Read the model definition and answer for the solid it produces. Units are mm, in the model's axes. A direction names the side the tool comes from. Give positions to 0.01 mm unless a question says otherwise; leave off trailing zeros. Write each loop counter-clockwise with the first axis right and the second up, starting at its lowest first coordinate (ties: lowest second). Pieces come first, ordered by that corner, then holes. Notation, with made-up numbers: M -28,20 L 5,20 A16 cw 5,49 Z; hole C 74,41 d3. An arc over 180 degrees is marked long. Use a Markdown table: item, result. Add a question column.
Item 1: A cutting plane is placed at A-A on x = -59.5. Determine the outline of the cut face in (y, z).
Item 2: For faces 1 (the flat face through (-43.365, -85.368, -12.86)), 2 (the cylindrical face through (-69.5, -93.5, -24.5)), determine the directions among +Z, -Z, +X, -X, +Y, -Y from which every point of the face is accessible in a straight line to the end or side of a thin tool.
Item 3: A cutting plane is placed at B-B on z = -5.75. Determine the outline of the cut face in (x, y), then the cut area to 3 significant figures.
Item 4: Consider probe 1 along Z at (x, y) = (-61, -96); probe 2 along Y at (x, z) = (-68.5, -18.25); probe 3 along Y at (x, z) = (-72, -5.25). Determine where each line is inside the solid, lowest interval first. Write a range as [from, to].
Item 5: A cutting plane is placed at C-C on y = -65.5. Determine the outline of the cut face in (x, z).
Item 6: Given P1, Ø6, axis at y = -72, z = -7, coming from the -X side; P2, Ø10, axis at x = -63.5, y = -90, coming from the +Z side; P3, Ø6, axis at x = -56.5, z = -17.5, coming from the -Y side; P4, Ø10, axis at x = -44, z = -18.5, coming from the -Y side, each flat-ended and moving along its own axis, determine where each tip first touches the part or whether it passes through.
Item 7: A cutting plane is placed at D-D on x = -68. Count the separate pieces of the cut face and the enclosed holes in it, then the cut area to 3 significant figures.
Item 8: The mould has two halves that part along Z. Classify faces 3 (the flat face through (-50, -90, -26)), 4 (the flat face through (-46.063, -70.681, -12.86)), 5 (the flat face through (-48.637, -69.14, -12.818)): pulls with the +Z half, pulls with the -Z half, needs draft (parallel to the pull), parting line crosses it, or undercut.
Autodesk Inventor part; units mm, degrees
ref_plane "YZ Plane" through (0, 0, 0) normal (1, 0, 0) x (0, 1, 0)
ref_plane "XZ Plane" through (0, 0, 0) normal (0, 1, 0) x (-1, 0, 0)
ref_plane "XY Plane" through (0, 0, 0) normal (0, 0, 1) x (1, 0, 0)
sketch "Sketch1" plane through (0, 0, 0) normal (0, 0, 1) x (1, 0, 0)
  circle A0 centre (-48.3826, -94.0192) radius 2.5
  circle A1 centre (2.8152, 8.6005) radius 2.5
  line L0 (-48.3826, -94.0192) -> (40.5013, 54.4144)
  line L1 (2.8152, 8.6005) -> (32.8522, -42.034)
  line L2 (-2.0828, 38.9998) -> (-2.0828, -39)
  line L3 (-2.0828, -0.0001) -> (69.8745, -0.0001)
  line L4 (7.9172, -0.0001) -> (-0.6834, -5.1021)
  line L5 (2.8152, 8.6005) -> (7.9172, -0.0001)
  line L6 (7.9172, -0.0001) -> (16.5177, 5.1019)
  line L7 (7.9172, -0.0001) -> (-0.6834, -5.1021)
  line L8 (-0.6834, -5.1021) -> (-0.6834, -5.1021)
  line L9 (7.9172, -0.0001) -> (16.5177, 5.1019)
  line L10 (16.5177, 5.1019) -> (16.5177, 5.1019)
  line L11 (7.9172, -0.0001) -> (-0.6622, 5.1374)
  line L12 (7.9172, -0.0001) -> (16.4966, -5.1375)
  line L13 (-48.3826, -94.0192) -> (-43.2452, -85.4397)
  line L14 (-54.6233, -56.9895) -> (-9.7188, -83.8789)
  line L15 (-43.2452, -85.4397) -> (-34.6657, -90.5772)
  line L16 (-43.2452, -85.4397) -> (-51.8246, -80.3023)
  line L17 (-34.6657, -90.5772) -> (16.4966, -5.1375)
  line L18 (-0.6622, 5.1374) -> (-51.8246, -80.3023)
  line L19 (-3.7386, 0) -> (13.452, 10.2217)
  line L20 (-3.7386, 0) -> (13.4203, -10.2749)
  circle A2 centre (6.9172, -34) radius 2.5
  circle A3 centre (6.9172, -34) radius 5
  circle A4 centre (6.9172, 34) radius 2.5
  circle A5 centre (6.9172, 34) radius 4.9998
  line L21 (15.8878, 38.9998) -> (-2.0828, 38.9998)
  line L22 (-2.0828, -39) -> (15.933, -39)
  line L23 (-13.3434, -16.0398) -> (19.6624, -35.8041)
  line L24 (-13.3434, 16.0396) -> (19.6624, 35.8039)
  line L25 (-13.3434, -16.0398) -> (-15.9172, -14.4985)
  line L26 (-2.0828, -0.0001) -> (-26.2435, -0.0001)
  line L27 (-15.9172, -14.4985) -> (-7.2354, -0.0001)
  line L28 (-13.3434, 16.0396) -> (-15.9172, 14.4984)
  line L29 (-15.9172, 14.4984) -> (-7.2354, -0.0001)
  line L30 (13.4203, -10.2749) -> (15.9172, -11.7701)
  line L31 (15.933, -39) -> (15.8878, 38.9998)
  line L32 (13.452, 10.2217) -> (15.9037, 11.6795)
  line L33 (15.9037, 11.6795) -> (6.3124, 27.8097)
  line L34 (15.9172, -11.7701) -> (6.3124, -27.8099)
  line L35 (15.9037, 11.6795) -> (15.9172, -11.7701)
  line L36 (-15.9172, -14.4985) -> (-15.9172, 14.4984)
  line L37 (6.3124, 27.8097) -> (-15.9172, 14.4984)
  circle A6 centre (-48.3826, -94.0192) radius 2.5
  line L38 (-311.4249, 0) -> (127.5863, 0)
  line L39 (-170.3704, -117.2696) -> (-13.4682, 154.4931)
  line L40 (-102.6648, 0) -> (-157.9558, -95.7668)
  line L41 (-157.9558, -95.7668) -> (-48.3826, -94.0192)
  line L42 (-48.3826, -94.0192) -> (-58.3814, -94.1786)
  line L43 (-58.3814, -94.1786) -> (-58.5408, -84.1799)
  line L44 (-58.5408, -84.1799) -> (-58.2219, -104.1774)
  line L45 (-51.8246, -80.3023) -> (-41.5497, -63.1434)
  line L46 (-41.5497, -63.1434) -> (-24.3908, -73.4184)
  line L47 (-58.5408, -84.1799) -> (-78.5383, -84.4989)
  line L48 (-78.5383, -84.4989) -> (-78.2193, -104.4963)
  line L49 (-78.2193, -104.4963) -> (-58.2219, -104.1774)
  line L50 (-58.5408, -84.1799) -> (-51.8246, -80.3023)
  line L51 (-58.2219, -104.1774) -> (-26.2433, -104.1774)
  line L52 (-34.6657, -90.5772) -> (-48.6317, -113.8999)
  circle A7 centre (-48.3828, -94.0194) radius 2.5
  point P0 (0, 0)
  point P1 (6.9172, -21)
  point P2 (-3.7386, 0)
  point P3 (-42.2878, -64.3761)
  point P4 (-42.8097, -104.1774)
  point P5 (-25.129, -74.6511)
  dimension "d0" = 10
  dimension "d1" = 10
  dimension "d2" = 10
  dimension "d3" = 10
  dimension "d4" = 10
  dimension "d5" = 10
  dimension "d6" = 10
  dimension "d7" = 10
  dimension "d8" = 10
  dimension "d9" = 10
  dimension "d10" = 10
  dimension "d11" = 20
  dimension "d12" = 20
  dimension "d13" = 3
  dimension "d14" = 3
  dimension "d20" = 110.582
  dimension "d21" = 10
  dimension "d22" = 10
  dimension "d23" = 20
  dimension "d24" = 20
  dimension "d25" = 20
  dimension "d26" = 121.827
  dimension "d27" = 146.9972
extrude "Extrusion1" add sketch "Sketch1" against normal blind 3 contours A0 L0 L15 L52 L51 L44 L41 | A0 L41 L43 L50 L16 L0 | L16 L18 L14 L0 | L0 L14 L17 L15 | L44 L49 L48 L41 | L41 L48 L47 L43
sketch "Sketch2" plane through (0, 0, -3) normal (0, 0, -1) x (-1, 0, 0)
  line L0 (51.8246, -80.3023) -> (42.2878, -64.3761)
  line L1 (25.129, -74.6511) -> (42.8097, -104.1774)
  line L2 (78.5383, -84.4989) -> (58.5408, -84.1799)
  line L3 (58.5408, -84.1799) -> (51.8246, -80.3023)
  line L4 (42.2878, -64.3761) -> (25.129, -74.6511)
  line L5 (78.5383, -84.4989) -> (78.2193, -104.4963)
  line L6 (58.5408, -84.1799) -> (58.5408, -81.1799)
  line L7 (51.8246, -80.3023) -> (54.3984, -78.761)
  line L8 (42.8097, -104.1774) -> (40.2359, -105.7186)
  line L9 (42.8097, -104.1774) -> (42.7827, -107.1772)
  line L10 (78.5383, -84.4989) -> (78.5383, -81.4989)
  line L11 (78.2193, -104.4963) -> (78.2193, -107.4963)
  line L12 (42.2878, -64.3761) -> (44.8616, -62.8349)
  line L13 (42.2878, -64.3761) -> (25.129, -74.6511)
  line L14 (25.129, -74.6511) -> (22.5551, -76.1923)
  line L15 (78.5383, -81.4989) -> (58.5408, -81.1799)
  line L16 (58.5408, -81.1799) -> (54.3984, -78.761)
  line L17 (54.3984, -78.761) -> (44.8616, -62.8349)
  line L18 (22.5551, -76.1923) -> (40.2359, -105.7186)
  line L19 (40.2359, -105.7186) -> (42.7827, -107.1772)
  line L20 (78.2193, -107.4963) -> (42.7827, -107.1772)
  line L21 (58.5408, -84.1799) -> (58.2219, -104.1774)
  line L22 (51.8246, -80.3023) -> (34.6657, -90.5772)
  circle A0 centre (48.3826, -94.0192) radius 2.5
  circle A1 centre (48.3826, -94.0192) radius 2.5
  line L23 (78.2193, -104.4963) -> (42.8097, -104.1774)
  line L24 (58.2219, -104.1774) -> (42.8097, -104.1774)
  line L25 (78.2193, -104.4963) -> (58.2219, -104.1774)
  point P0 (0, 0)
  dimension "d30" = 3
  dimension "d31" = 3
  dimension "d32" = 3
  dimension "d33" = 3
  dimension "d34" = 3
  dimension "d35" = 3
  dimension "d36" = 3
  dimension "d37" = 3
extrude "Extrusion2" add sketch "Sketch2" along normal blind 20 and the other way blind 3 contours L7 L16 L6 L3 | L0 L12 L17 L7 | L6 L15 L10 L2 | L1 L8 L18 L14 | L25 L23 L24 | L9 L19 L8 | L23 L11 L20 L9
sketch "Sketch3" plane through (0, 0, -3) normal (0, 0, -1) x (-1, 0, 0)
  line L0 (58.5408, -84.1799) -> (51.8246, -80.3023)
  line L1 (51.8246, -80.3023) -> (34.6657, -90.5772)
  line L2 (25.129, -74.6511) -> (42.8097, -104.1774)
  line L3 (42.8097, -104.1774) -> (58.2219, -104.1774)
  line L4 (58.5408, -84.1799) -> (58.2219, -104.1774)
  line L5 (78.2193, -104.4963) -> (42.8097, -104.1774)
  line L6 (42.8097, -104.1774) -> (25.129, -74.6511)
  circle A0 centre (48.3828, -94.0194) radius 2.5
  point P0 (0, 0)
  dimension "d42" = 119.086
extrude "Extrusion3" add sketch "Sketch3" along normal blind 20
sketch "Sketch4" plane through (0, 0, -23) normal (0, 0, -1) x (-1, 0, 0)
  point P0 (0, 0)
sketch "Sketch5" plane through (0, 0, -23) normal (0, 0, -1) x (-1, 0, 0)
  circle A0 centre (48.3828, -94.0194) radius 2.5
  line L0 (44.8616, -62.8349) -> (42.2878, -64.3761)
  line L1 (42.2878, -64.3761) -> (51.8246, -80.3023)
  line L2 (51.8246, -80.3023) -> (34.6657, -90.5772)
  line L3 (34.6657, -90.5772) -> (25.129, -74.6511)
  line L4 (25.129, -74.6511) -> (22.5551, -76.1923)
  line L5 (22.5551, -76.1923) -> (40.2359, -105.7186)
  line L6 (40.2359, -105.7186) -> (42.7827, -107.1772)
  line L7 (42.7827, -107.1772) -> (78.2193, -107.4963)
  line L8 (78.2193, -107.4963) -> (78.2193, -104.4963)
  line L9 (78.2193, -104.4963) -> (58.2219, -104.1774)
  line L10 (58.2219, -104.1774) -> (58.5408, -84.1799)
  line L11 (58.5408, -84.1799) -> (78.5383, -84.4989)
  line L12 (78.5383, -84.4989) -> (78.5383, -81.4989)
  line L13 (78.5383, -81.4989) -> (58.5408, -81.1799)
  line L14 (58.5408, -81.1799) -> (54.3984, -78.761)
  line L15 (54.3984, -78.761) -> (44.8616, -62.8349)
  line L16 (58.5408, -84.1799) -> (58.2219, -104.1774)
  line L17 (58.2219, -104.1774) -> (78.2193, -104.4963)
  line L18 (78.2193, -104.4963) -> (78.5383, -84.4989)
  line L19 (78.5383, -84.4989) -> (58.5408, -84.1799)
  line L20 (34.6657, -90.5772) -> (51.8246, -80.3023)
  line L21 (51.8246, -80.3023) -> (42.2878, -64.3761)
  line L22 (42.2878, -64.3761) -> (25.129, -74.6511)
  line L23 (25.129, -74.6511) -> (34.6657, -90.5772)
  point P0 (0, 0)
extrude "Extrusion4" add sketch "Sketch5" along normal blind 3
sketch "Sketch6" plane through (0, 0, 0) normal (0, 0, 1) x (1, 0, 0)
  line L0 (-42.2878, -64.3761) -> (-25.129, -74.6511)
  line L1 (-33.7084, -69.5136) -> (-49.5228, -95.9232)
  line L2 (-33.7084, -69.5136) -> (-38.8459, -78.093)
  circle A0 centre (-38.8459, -78.093) radius 1.5
  line L3 (-78.5383, -84.4989) -> (-78.2193, -104.4963)
  line L4 (-78.3788, -94.4976) -> (-68.3788, -94.4976)
  circle A1 centre (-68.3788, -94.4976) radius 1.5
  point P0 (0, 0)
  dimension "d47" = 10
  dimension "d48" = 3
  dimension "d56" = 10
  dimension "d57" = 3
extrude "Extrusion5" cut sketch "Sketch6" against normal through all
sketch "Sketch7" plane through (-44.8616, -62.8349, -26) normal (-0.857942, 0.5137465, 0) x (0, 0, 1)
  line L0 (0, 0) -> (26, 0)
  line L1 (26, 0) -> (13, 0)
  line L2 (13, 0) -> (13, -10)
  line L3 (13, -10) -> (26, -10)
  line L4 (26, -10) -> (26, 0)
  circle A0 centre (13, -10) radius 1.5
  point P0 (26, 76.9562)
  dimension "d51" = 13
  dimension "d52" = 10
  dimension "d53" = 3
extrude "Extrusion6" cut sketch "Sketch7" against normal through all contours A0 L3 L2 | L2 L3 A0
sketch "Sketch8" plane through (-58.5408, -81.1799, 0) normal (-0.0159478, 0.9998728, 0) x (0.9998728, 0.0159478, 0)
  line L0 (-20.0478, 3) -> (-20.0478, 23)
  line L1 (-20.0478, 13) -> (-10.0478, 13)
  circle A0 centre (-10.0478, 13) radius 1.5
  point P0 (59.828, 0)
  dimension "d58" = 10
  dimension "d59" = 3
extrude "Extrusion7" cut sketch "Sketch8" against normal through all
properties part number "2020_nodes_conn"
Filled in:
| question | item | result |
|---|---|---|
| 1 | outline | M -107.33,-26 L -81.2,-26 L -81.2,0 L -107.33,0 Z; hole M -104.2,-23 L -84.2,-23 L -84.2,-3 L -104.2,-3 Z |
| 2 | face 1 | none |
| 2 | face 2 | +Z, -Z |
| 3 | outline | M -78.54,-84.5 L -58.54,-84.18 L -58.22,-104.18 L -78.22,-104.5 L -78.22,-107.5 L -42.78,-107.18 L -40.24,-105.72 L -22.56,-76.19 L -25.13,-74.65 L -34.67,-90.58 L -51.82,-80.3 L -42.29,-64.38 L -44.86,-62.83 L -54.4,-78.76 L -58.54,-81.18 L -78.54,-81.5 Z; hole C -48.38,-94.02 d5 |
| 3 | area | 739 mm² |
| 4 | probe 1 | [-26, -23], [-3, 0] |
| 4 | probe 2 | [-107.41, -104.34], [-84.34, -81.34] |
| 4 | probe 3 | [-107.44, -104.4], [-84.39, -81.39] |
| 5 | outline | M -46.46,-26 L -40.41,-26 L -40.41,-23 L -42.96,-23 L -42.96,-3 L -40.41,-3 L -40.41,0 L -46.46,0 Z |
| 6 | P1 | x = -52.15 |
| 6 | P2 | z = 0 |
| 6 | P3 | y = -107.33 |
| 6 | P4 | y = -107.23 |
| 7 | separate pieces | 4 |
| 7 | enclosed holes | 0 |
| 7 | area | 243 mm² |
| 8 | face 3 | pulls with the -Z half |
| 8 | face 4 | undercut |
| 8 | face 5 | needs draft |
